from build123d import *

# Parameters (mm, degrees)
BOSS_EXTRUDE1_DEPTH = 10
SKETCH2_W           = 7.883034156
SKETCH2_H           = 11.550106774
CUT_EXTRUDE1_DEPTH  = 5
SKETCH3_R           = 2.5
CUT_EXTRUDE2_DEPTH  = 3


with BuildPart() as part:
    # Sketch1 → Boss-Extrude1 (new body)
    with BuildSketch(Plane.XY):
        Polygon((2.5, -30), (2.5, -32.5), (7, -32.5), (7, -35), (0, -35), (0, -32.5), (0, -2.5), (0, 0), (110, 0), (110, -2.5), (110, -32.5), (110, -35), (103, -35), (103, -32.5), (107.5, -32.5), (107.5, -30), (103, -30), (103, -27.5), (107.5, -27.5), (107.5, -2.5), (2.5, -2.5), (2.5, -27.5), (7, -27.5), (7, -30), align=None)
    extrude(amount=BOSS_EXTRUDE1_DEPTH)

    # Sketch2 → Cut-Extrude1 (cut)
    with BuildSketch(Plane.XY.offset(10)):
        with Locations((3.941517078, -29.224946613)):
            Rectangle(SKETCH2_W, SKETCH2_H)
    extrude(amount=-CUT_EXTRUDE1_DEPTH, mode=Mode.SUBTRACT)

    # Sketch3 → Cut-Extrude2 (cut)
    with BuildSketch(Plane(origin=(0, 0, 0), x_dir=(1, 0, 0), z_dir=(0, 1, 0))):
        with Locations((98, -5)):
            Circle(SKETCH3_R)
        with Locations((28, -5)):
            Circle(SKETCH3_R)
    extrude(amount=-CUT_EXTRUDE2_DEPTH, mode=Mode.SUBTRACT)


solid = part.part
Work out the finished part from the listing and answer in its coordinate system (mm). A direction names the side the tool comes from. Give positions to 0.01 mm unless a question says otherwise; leave off trailing zeros. Order: outer loops, then holes, each group sorted by start corner. A loop starts at its lowest first (then second) coordinate and runs counter-clockwise, first axis right, second up. Notation, with made-up numbers: (-23.75, 49.25) -> (17.25, 49.25) arc R18 ccw to (17.25, 55.25) -> close; hole circle Ø3 at (9, 51). An arc over 180 degrees is marked (long way). Answer as a JSON object with one key per item and string values. Group by question number.
1. Section C-C on z = 6.25 is taken. Determine the outline of the cut face in (x, y).
2. Section D-D on x = 82 is taken. Determine the outline of the cut face in (y, z), plus the area to 3 significant figures.
3. Section B-B on x = 98 is taken. Determine the outline of the cut face in (y, z).
4. Flat-ended cylindrical pins translate along their axes: pin 1 Ø3.5 at (x, y) = (4.5, -27) entering from +Z; pin 2 Ø1 at (x, z) = (30.5, 7) entering from -Y; pin 3 Ø0.8 at (y, z) = (-28.5, 7) entering from -X. Find the tip coordinate at first contact, or state that the pin passes through.
5. Section A-A on y = -12.5 is taken. Determine the outline of the cut face in (x, z), plus the area to 3 significant figures.
6. A tool of negligible diameter and unlimited length cuts with its end or side. For faces 5 (the flat face through (103, -29, 5)), 6 (the flat face through (1, -23.45, 8)), 7 (the flat face through (105, -30, 5)), 8 (the flat face through (4, -35, 2)), from which of +Z, -Z, +X, -X, +Y, -Y can it reach the whole face along a straight path? Write none if from no direction.
7. The mould has two halves that part along X. Classify faces 1 (the flat face through (2.5, -15, 5)), 2 (the flat face through (0, -13, 5)), 3 (the flat face through (107, -35, 5)), 4 (the flat face through (110, -18, 5)): released by +X, released by -X, zero draft, split by the parting line, or undercut.
8. Consider line 1 along X through (y, z) = (-0.5, 5); line 2 along X through (y, z) = (-3.5, 3.75); line 3 along Z through (x, y) = (28, -1.25). Determine where each line is inside the solid, lowest interval first. Write a range as [from, to].
Result sheet:
{
 "1": {"outline": "(0, -23.45) -> (2.5, -23.45) -> (2.5, -2.5) -> (25.83, -2.5) -> (25.83, 0) -> (0, 0) -> close; (30.17, -2.5) -> (95.83, -2.5) -> (95.83, 0) -> (30.17, 0) -> close; (100.17, -2.5) -> (107.5, -2.5) -> (107.5, -27.5) -> (103, -27.5) -> (103, -30) -> (107.5, -30) -> (107.5, -32.5) -> (103, -32.5) -> (103, -35) -> (110, -35) -> (110, 0) -> (100.17, 0) -> close"},
 "2": {"outline": "(-2.5, 0) -> (0, 0) -> (0, 10) -> (-2.5, 10) -> close", "area": "25.0 mm^2"},
 "3": {"outline": "(-2.5, 0) -> (0, 0) -> (0, 2.5) -> (-2.5, 2.5) -> close; (-2.5, 7.5) -> (0, 7.5) -> (0, 10) -> (-2.5, 10) -> close"},
 "4": {"pin 1": "stops at z = 5", "pin 2": "stops at y = -2.5", "pin 3": "stops at x = 103"},
 "5": {"outline": "(0, 0) -> (2.5, 0) -> (2.5, 10) -> (0, 10) -> close; (107.5, 0) -> (110, 0) -> (110, 10) -> (107.5, 10) -> close", "area": "50.0 mm^2"},
 "6": {"face 5": "+Z, -Z, -Y", "face 6": "+Z, -X, -Y", "face 7": "+Z, -Z", "face 8": "+Z, -Z, +X, -X, -Y"},
 "7": {"face 1": "undercut", "face 2": "released by -X", "face 3": "zero draft", "face 4": "released by +X"},
 "8": {"line 1": "x = [0, 25.5], [30.5, 95.5], [100.5, 110]", "line 2": "x = [0, 2.5], [107.5, 110]", "line 3": "z = [0, 2.5], [7.5, 10]"}
}
